Could you check a few things on this model? Use its own coordinates, in mm. A direction names the side the tool comes from. Coordinates: 2 decimals unless noted, no trailing zeros. Order: outer loops, then holes, each group sorted by start corner. A loop starts at its lowest first (then second) coordinate and runs counter-clockwise, first axis right, second up. Notation, with made-up numbers: (47, 84.5) -> (57, 84.5) arc R19 cw to (57, 109.5) -> close; hole circle Ø10 at (29, 15.5). An arc over 180 degrees is marked (long way). Put each result on its own line as item: value. Start each with the question number.
Q1. We'd pull the mould along Z, two halves only. Please class faces 3 (the face through (56.515, 0, 0)), 4 (the face through (25.595, -0.099, -15.255)), 5 (the face through (3.345, -2.93, 22.313)): +Z half, -Z half, draft (parallel to the pull), parting line (faces both ways), or undercut.
Q2. For faces 1 (the face through (51.918, 19, -2)), 2 (the face through (25.6, -15.51, -1.04)), which set-ups out of +Z, -Z, +X, -X, +Y, -Y let a thin tool reach every point of the face, with its end or its side?
Q3. If we section it at B-B (x = 9): Please give me the cut outline in (y, z).
Q4. Please list where these lines run through material, in increasing order: line 1 along Z through (x, y) = (17, 0); line 2 along Y through (x, z) = (27, 0.5); line 3 along Z through (x, y) = (49.5, 12.5).
Q5. Will these pins go through, and if not, where does the flat tip stop? pin 1 (8 mm diameter, centred on y = -5, z = -14.5, fed in from -X); pin 2 (2 mm diameter, centred on x = 36, y = -17.5, fed in from +Z); pin 3 (10 mm diameter, centred on x = 11.5, y = 7.5, fed in from -Z); pin 4 (8 mm diameter, centred on x = 40.5, y = -11.5, fed in from +Z).
Q6. If we section it at A-A (z = 0): Count the separate pieces of the cut face and the enclosed holes in it, and give its area (3 significant figures).
Autodesk Inventor part; units mm, degrees
ref_plane "YZ Plane" through (0, 0, 0) normal (1, 0, 0) x (0, 1, 0)
ref_plane "XZ Plane" through (0, 0, 0) normal (0, 1, 0) x (-1, 0, 0)
ref_plane "XY Plane" through (0, 0, 0) normal (0, 0, 1) x (1, 0, 0)
sketch "Sketch1" plane through (0, 0, 0) normal (0, 0, 1) x (1, 0, 0)
  line L0 (0, 0) -> (0, 22.5044)
  line L1 (0, 22.5044) -> (6.35, 22.5044)
  line L2 (6.35, 22.5044) -> (6.35, 19.9644)
  line L3 (6.35, 19.9644) -> (50.165, 19.9644)
  line L4 (50.165, 19.9644) -> (50.165, 22.5044)
  line L5 (50.165, 22.5044) -> (56.515, 22.5044)
  line L6 (56.515, 22.5044) -> (56.515, 0)
  line L7 (0, 0) -> (56.515, 0)
  dimension "d0" = 22.5044
  dimension "d1" = 6.35
  dimension "d2" = 2.54
  dimension "d3" = 43.815
  dimension "d4" = 6.35
revolve "Revolution1" add sketch "Sketch1" angle 360 about axis through (0, 0, 0) along (1, 0, 0)
sketch "Sketch2" plane through (0, 0, 0) normal (0, 0, 1) x (1, 0, 0)
  line L0 (6.35, 19.9644) -> (50.165, 19.9644)
  line L1 (6.35, -22.5044) -> (6.35, 22.5044)
  line L2 (50.165, -22.5044) -> (50.165, 22.5044)
  line L3 (6.3525, 22.5044) -> (50.1625, 22.5044)
  line L4 (6.3525, 22.5044) -> (6.3525, 19.9644)
  line L5 (50.1625, 22.5044) -> (50.1625, 19.9644)
  line L6 (-11.303, 0) -> (67.818, 0)
  point P0 (0, 0)
  dimension "d6" = 0.0025
  dimension "d7" = 0.0025
revolve "Revolution2" add sketch "Sketch2" angle 360 about axis through (-10, 0, 0) along (1, 0, 0) contours L4 L3 L5 L0
chamfer "Chamfer1" distance 0.254 angle 45 2 edges at (56.515, -22.5044, 0) (0, -22.5044, 0)
sketch "Sketch3" plane through (56.515, 0, 0) normal (1, 0, 0) x (0, 0, -1)
  circle A0 centre (0, 0) radius 22.2504
  circle A1 centre (0, 0) radius 17.5006 construction
  line L0 (0, 0) -> (-12.3748, 12.3748) construction
  line L1 (0, 0) -> (-17.5006, 0) construction
  point P0 (0, 17.5006)
  point P1 (0, -17.5006)
  point P2 (17.5006, 0)
  dimension "d12" = 17.5006
  dimension "d14" = 45
hole "Hole1" at (56.515, 17.5006, 0) at (56.515, -17.5006, 0) at (56.515, 0, 17.5006) at (56.515, 0, -17.5006) direction (-1, 0, 0) diameter 4.4958 end through all counterbore diameter 8.001 counterbore depth 4.5974
hole "Hole2" at (56.515, 12.3748, 12.3748) direction (-1, 0, 0) diameter 3.2512 depth 9 tip angle 118
pattern_circular "Circular Pattern1" count 4 over 360 about axis through (-10, 0, 0) along (1, 0, 0) of "Hole2"
equation "\"d7\" = d6"
properties part number "MOT_Gearbox_am0939" material "Steel, Mild"
The answers:
1. face 3: draft
1. face 4: undercut
1. face 5: parting line
2. face 1: +X
2. face 2: +X, -X
3. outline: circle Ø45.01 at (0, 0); hole circle Ø4.5 at (-17.5, 0); hole circle Ø4.5 at (0, -17.5); hole circle Ø4.5 at (0, 17.5); hole circle Ø4.5 at (17.5, 0)
4. line 1: -22.5 to -19.75, -15.25 to 15.25, 19.75 to 22.5
4. line 2: -22.5 to -19.69, -15.31 to 15.31, 19.69 to 22.5
4. line 3: -18.71 to -14, -10.75 to 10.75, 14 to 18.71
5. pin 1: x = 0
5. pin 2: z = 15.3
5. pin 3: z = -22.37
5. pin 4: z = 21.22
6. separate pieces: 3
6. enclosed holes: 0
6. area: 2,000 mm^2
